Part print with two shaded views. Sizes in mm from the minimum x, y, z corner. A direction names the side the tool comes from. Give positions to 0.01 mm unless a question says otherwise; leave off trailing zeros. Write each loop counter-clockwise with the first axis right and the second up, starting at its lowest first coordinate (ties: lowest second). Pieces come first, ordered by that corner, then holes. Notation, with made-up numbers: (-15, 52) -> (27, 52) arc R12 ccw to (27, 68) -> close; hole circle Ø5 at (-10.75, 5). An arc over 180 degrees is marked (long way). Answer as a JSON object with one key per item and string values.
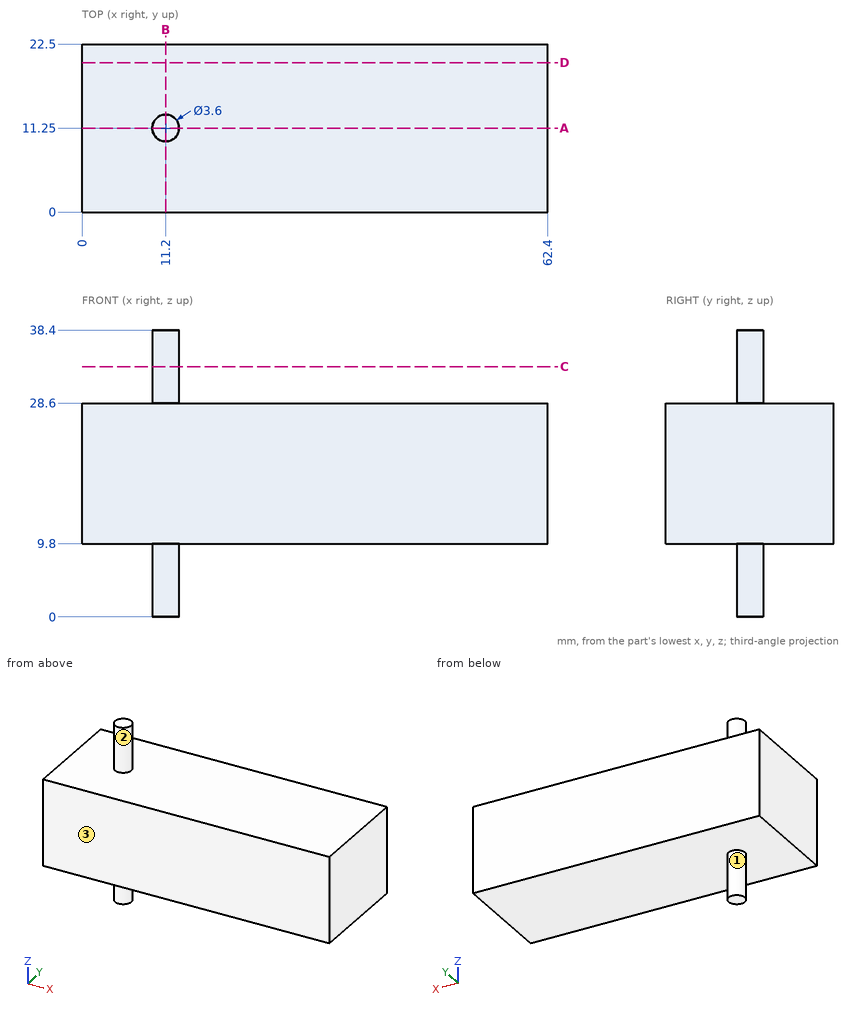
1) Slice it at B-B (x = 11.2). List the corners of the cut face in (y, z).
Model answer:
{"outline": "(0, 9.8) -> (9.45, 9.8) -> (9.45, 0) -> (13.05, 0) -> (13.05, 9.8) -> (22.5, 9.8) -> (22.5, 28.6) -> (13.05, 28.6) -> (13.05, 38.4) -> (9.45, 38.4) -> (9.45, 28.6) -> (0, 28.6) -> close"}
2) Pin check, flat tips, straight feed: pin 1 (7 mm diameter, centred on x = 36.5, y = 16, fed in from +Z); pin 2 (6 mm diameter, centred on y = 9, z = 33, fed in from +X); pin 3 (3 mm diameter, centred on x = 29, y = 11, fed in from -Z). Stop position of each tip, or through.
Model answer:
{"pin 1": "stops at z = 28.6", "pin 2": "stops at x = 13", "pin 3": "stops at z = 9.8"}
3) Slice it at D-D (y = 20). List the corners of the cut face in (x, z).
Model answer:
{"outline": "(0, 9.8) -> (62.4, 9.8) -> (62.4, 28.6) -> (0, 28.6) -> close"}
4) Slice it at C-C (z = 33.5). List the corners of the cut face in (x, y), then the cut area to 3 significant figures.
Model answer:
{"outline": "circle Ø3.6 at (11.2, 11.25)", "area": "10.2 mm2"}
5) 3-axis set-ups, long thin cutter, end or side, ignore diameter. For the marked faces 1, 2 and 3: which of +Z, -Z, +X, -X, +Y, -Y reach the whole face in a straight line?
Model answer:
{"face 1": "-Z", "face 2": "+Z", "face 3": "+Z, -Z, +X, -X, -Y"}
6) Slice it at A-A (y = 11.25). List the corners of the cut face in (x, z).
Model answer:
{"outline": "(0, 9.8) -> (9.4, 9.8) -> (9.4, 0) -> (13, 0) -> (13, 9.8) -> (62.4, 9.8) -> (62.4, 28.6) -> (13, 28.6) -> (13, 38.4) -> (9.4, 38.4) -> (9.4, 28.6) -> (0, 28.6) -> close"}
7) Wall check: probe 1 along Z at (x, y) = (48, 19.5); probe 2 along X at (y, z) = (11.25, 2); probe 3 along X at (y, z) = (10.25, 34). Give the ranges that are in metal, low to high.
Model answer:
{"probe 1": "z = 9.8 to 28.6", "probe 2": "x = 9.4 to 13", "probe 3": "x = 9.7 to 12.7"}
